Answer from the drawing. Dimensions are ordinates in mm from the lowest x, y and z of the part. Coordinates: 2 decimals unless noted, no trailing zeros. Loops run counter-clockwise (first coordinate to the right, second up) from the corner with the lowest first, then second, coordinate; pieces in that order, holes last. Notation, with made-up numbers: M 38,17.5 L 59,17.5 A32 ccw 59,43.5 Z; hole C -35,31 d2. An arc over 180 degrees is marked long. Put each result on its own line as item: value.
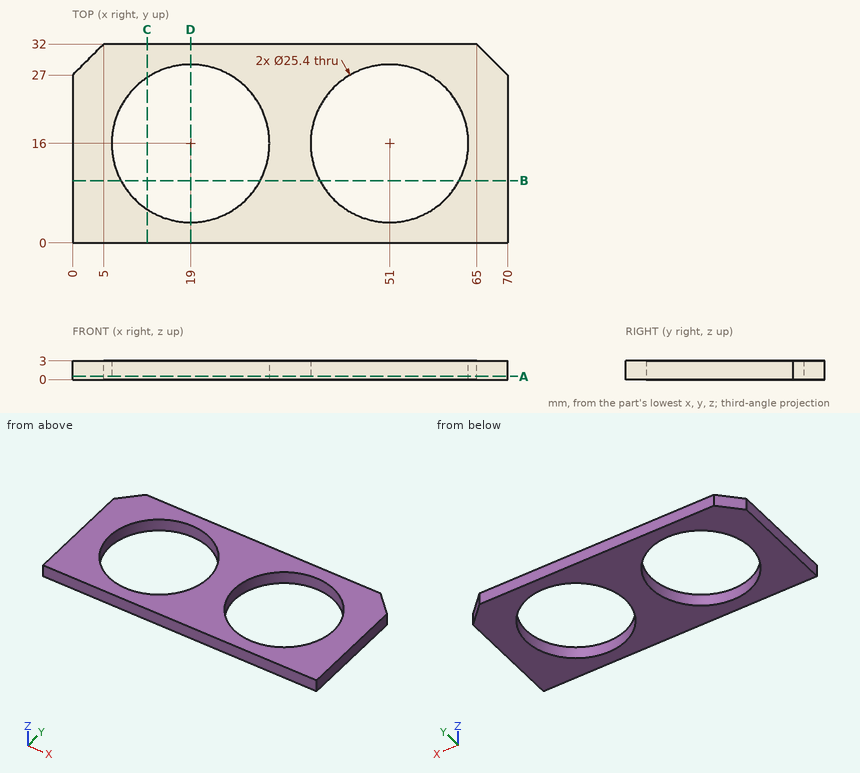
1) Straight lines are drawn through the part: line 1 (X direction, y = 8, z = 0.2); line 2 (Y direction, x = 51, z = 1.35); line 3 (X direction, y = 5.5, z = 1.8). For each, find the intervals that lie inside material, in ascending order. Write a range as [from, to].
Answer list:
line 1: x = [0, 9.14], [28.86, 41.14], [60.86, 70]
line 2: y = [0, 3.3], [28.7, 32]
line 3: x = [0, 11.86], [26.14, 43.86], [58.14, 70]
2) Find section C-C, the plane x = 12. Write down the section's boundary in (y, z), plus the area to 3 significant figures.
Answer list:
outline: M 0,0 L 5.4,0 L 5.4,3 L 0,3 Z; M 26.6,0 L 32,0 L 32,3 L 26.6,3 Z
area: 32.4 mm^2
3) Find section A-A, the plane z = 0.5. Write down the section's boundary in (x, y), plus the area to 3 significant figures.
Answer list:
outline: M 0,0 L 70,0 L 70,27 L 65,32 L 5,32 L 0,27 Z; hole C 19,16 d25.4; hole C 51,16 d25.4
area: 1,200 mm^2
4) Find section B-B, the plane y = 10. Write down the section's boundary in (x, z).
Answer list:
outline: M 0,0 L 7.81,0 L 7.81,3 L 0,3 Z; M 30.19,0 L 39.81,0 L 39.81,3 L 30.19,3 Z; M 62.19,0 L 70,0 L 70,3 L 62.19,3 Z
5) Given pin 1 Ø1.5 at (y, z) = (10.5, 2.5) entering from -X, flat-ended and moving along its own axis, determine where the tip first touches the part or whether it passes through.
Answer list:
pin 1: stops at x = 0
6) Find section D-D, the plane x = 19. Write down the section's boundary in (y, z).
Answer list:
outline: M 0,0 L 3.3,0 L 3.3,3 L 0,3 Z; M 28.7,0 L 32,0 L 32,3 L 28.7,3 Z
